Input: part model. Units: mm. Frame: model coordinates. A direction names the side the tool comes from. Give positions to 0.01 mm unless a question says otherwise; leave off trailing zeros. Write each loop counter-clockwise with the first axis right and the second up, starting at its lowest first coordinate (ties: lowest second). Pieces come first, ordered by that corner, then holes.
```python
from build123d import *

# Parameters (mm, degrees)
F1_DEPTH = 2


with BuildPart() as f1:
    # F0 (on Front) → F1 (new body)
    with BuildSketch(Plane.XZ):
        Polygon((-15.24, 12.7), (-15.24, -12.7), (15.24, -12.7), (15.24, 12.7), (11.58875, 12.7), (11.58875, 9.2292314502), (6.46642, 9.2292314502), (6.46642, 12.7), align=None)
        with BuildLine():
            Line((-11.641663, -5.17525), (-10.847913, -4.3815))
            Line((-10.847913, -4.3815), (-7.31308, -4.3815))
            ThreePointArc((-7.31308, -4.3815), (-6.7518139924, -4.6139839924), (-6.51933, -5.17525))
            Line((-6.51933, -5.17525), (-6.51933, -8.763))
            Line((-6.51933, -8.763), (-7.31308, -9.55675))
            Line((-7.31308, -9.55675), (-10.847913, -9.55675))
            Line((-10.847913, -9.55675), (-11.641663, -8.763))
            Line((-11.641663, -8.763), (-11.641663, -5.17525))
        make_face(mode=Mode.SUBTRACT)
        with BuildLine():
            add(Edge.make_bspline(
                [(0.005281, -5.969), (0.300451, -5.969), (0.539736, -5.729716), (0.539736, -5.434542)],
                knots=[0, 0, 0, 0, 1, 1, 1, 1], degree=3))
            add(Edge.make_bspline(
                [(-0.529178, -5.434542), (-0.529178, -5.729716), (-0.289893, -5.969), (0.005281, -5.969)],
                knots=[0, 0, 0, 0, 1, 1, 1, 1], degree=3))
            add(Edge.make_bspline(
                [(0.005281, -4.900084), (-0.289893, -4.900084), (-0.529178, -5.139369), (-0.529178, -5.434542)],
                knots=[0, 0, 0, 0, 1, 1, 1, 1], degree=3))
            add(Edge.make_bspline(
                [(0.539736, -5.434542), (0.539736, -5.139369), (0.300451, -4.900084), (0.005281, -4.900084)],
                knots=[0, 0, 0, 0, 1, 1, 1, 1], degree=3))
        make_face(mode=Mode.SUBTRACT)
        with BuildLine():
            add(Edge.make_bspline(
                [(-7.868719, -0.296334), (-7.427422, -0.296334), (-7.069678, 0.061408), (-7.069678, 0.502708)],
                knots=[0, 0, 0, 0, 1, 1, 1, 1], degree=3))
            add(Edge.make_bspline(
                [(-8.667764, 0.502708), (-8.667764, 0.061408), (-8.310019, -0.296334), (-7.868719, -0.296334)],
                knots=[0, 0, 0, 0, 1, 1, 1, 1], degree=3))
            add(Edge.make_bspline(
                [(-7.868719, 1.30175), (-8.310019, 1.30175), (-8.667764, 0.944007), (-8.667764, 0.502708)],
                knots=[0, 0, 0, 0, 1, 1, 1, 1], degree=3))
            add(Edge.make_bspline(
                [(-7.069678, 0.502708), (-7.069678, 0.944007), (-7.427422, 1.30175), (-7.868719, 1.30175)],
                knots=[0, 0, 0, 0, 1, 1, 1, 1], degree=3))
        make_face(mode=Mode.SUBTRACT)
        with BuildLine():
            add(Edge.make_bspline(
                [(0.005281, -2.550584), (1.761708, -2.550584), (3.185572, -1.126719), (3.185572, 0.629708)],
                knots=[0, 0, 0, 0, 1, 1, 1, 1], degree=3))
            add(Edge.make_bspline(
                [(-3.175014, 0.629708), (-3.175014, -1.126719), (-1.751146, -2.550584), (0.005281, -2.550584)],
                knots=[0, 0, 0, 0, 1, 1, 1, 1], degree=3))
            add(Edge.make_bspline(
                [(0.005281, 3.81), (-1.751146, 3.81), (-3.175014, 2.386135), (-3.175014, 0.629708)],
                knots=[0, 0, 0, 0, 1, 1, 1, 1], degree=3))
            add(Edge.make_bspline(
                [(3.185572, 0.629708), (3.185572, 2.386135), (1.761708, 3.81), (0.005281, 3.81)],
                knots=[0, 0, 0, 0, 1, 1, 1, 1], degree=3))
        make_face(mode=Mode.SUBTRACT)
        with BuildLine():
            add(Edge.make_bspline(
                [(7.889861, -0.296334), (8.331161, -0.296334), (8.688906, 0.061408), (8.688906, 0.502708)],
                knots=[0, 0, 0, 0, 1, 1, 1, 1], degree=3))
            add(Edge.make_bspline(
                [(7.090822, 0.502708), (7.090822, 0.061408), (7.448564, -0.296334), (7.889861, -0.296334)],
                knots=[0, 0, 0, 0, 1, 1, 1, 1], degree=3))
            add(Edge.make_bspline(
                [(7.889861, 1.30175), (7.448564, 1.30175), (7.090822, 0.944007), (7.090822, 0.502708)],
                knots=[0, 0, 0, 0, 1, 1, 1, 1], degree=3))
            add(Edge.make_bspline(
                [(8.688906, 0.502708), (8.688906, 0.944007), (8.331161, 1.30175), (7.889861, 1.30175)],
                knots=[0, 0, 0, 0, 1, 1, 1, 1], degree=3))
        make_face(mode=Mode.SUBTRACT)
        with BuildLine():
            add(Edge.make_bspline(
                [(0.005281, 6.148916), (0.300451, 6.148916), (0.539736, 6.388201), (0.539736, 6.683375)],
                knots=[0, 0, 0, 0, 1, 1, 1, 1], degree=3))
            add(Edge.make_bspline(
                [(-0.529178, 6.683375), (-0.529178, 6.388201), (-0.289893, 6.148916), (0.005281, 6.148916)],
                knots=[0, 0, 0, 0, 1, 1, 1, 1], degree=3))
            add(Edge.make_bspline(
                [(0.005281, 7.217833), (-0.289893, 7.217833), (-0.529178, 6.978548), (-0.529178, 6.683375)],
                knots=[0, 0, 0, 0, 1, 1, 1, 1], degree=3))
            add(Edge.make_bspline(
                [(0.539736, 6.683375), (0.539736, 6.978548), (0.300451, 7.217833), (0.005281, 7.217833)],
                knots=[0, 0, 0, 0, 1, 1, 1, 1], degree=3))
        make_face(mode=Mode.SUBTRACT)
    extrude(amount=F1_DEPTH)


solid = f1.part
```
Q1. Section B-B, the plane y = -1.5. Give the number of separate pieces and of enclosed holes in the cut face, then the cut area to 3 significant figures.
Q2. Section C-C, the plane x = 10.5. Return the cut outline in (y, z), then the cut area to 3 significant figures.
Q3. Material intervals for line 1 along X through (y, z) = (-0.55, 0.5); line 2 along X through (y, z) = (-1.1, 11.75); line 3 along Z through (x, y) = (-7.5, -0.55), sorted ascending.
Q4. Mould query, pull axis X, two halves, no side actions, for faces 4 (the flat face through (-15.24, -1, 0)), 5 (the flat face through (13, -1, 12.7)), 6 (the flat face through (-9, -1, -9.557)). Classes: +X half, -X half, draft (parallel to the pull), parting line (faces both ways), or undercut.
Q5. Section A-A, the plane z = -7.5. Return the cut outline in (x, y), then the cut area to 3 significant figures.
Q6. Access query for faces 1 (the flat face through (-9, -1, -4.382)), 2 (the flat face through (0, -2, -3)), 3 (the flat face through (6.466, -1, 11)). Directions: +Z, -Z, +X, -X, +Y, -Y. A direction counts if a zero-diameter tool reaches every point of the face in a straight line with its end or side. Return the directions, or none.
Solutions:
1. separate pieces: 1
1. enclosed holes: 6
1. area: 693 mm2
2. outline: (-2, -12.7) - (0, -12.7) - (0, 9.23) - (-2, 9.23) - close
2. area: 43.9 mm2
3. line 1: x = -15.24 to -8.67, -7.07 to -3.17, 3.18 to 7.09, 8.69 to 15.24
3. line 2: x = -15.24 to 6.47, 11.59 to 15.24
3. line 3: z = -12.7 to -9.56, -4.38 to -0.21, 1.21 to 12.7
4. face 4: -X half
4. face 5: draft
4. face 6: undercut
5. outline: (-15.24, -2) - (-11.64, -2) - (-11.64, 0) - (-15.24, 0) - close; (-6.52, -2) - (15.24, -2) - (15.24, 0) - (-6.52, 0) - close
5. area: 50.7 mm2
6. face 1: +Y, -Y
6. face 2: +Z, -Z, +X, -X, -Y
6. face 3: +Z, +Y, -Y
